Could you check a few things on this model? Use its own coordinates, in mm. Face numbers are marked on the shaded views. A direction names the side the tool comes from. Coordinates: 2 decimals unless noted, no trailing zeros. Loops run counter-clockwise (first coordinate to the right, second up) from the corner with the lowest first, then second, coordinate; pieces in that order, holes last.
1) Will this pin go through, and if not, where does the flat tip stop? P1, Ø7, axis at x = -38.5, z = -14, coming from the -Y side.
2) If I drill on line 1 along Z through (x, y) = (-44, 24); line 2 along X through (y, z) = (10, -19); line 3 along X through (y, z) = (12, 15.5), over which ranges is the centre line in solid material (lowest first)?
3) Imagine slicing it at B-B on y = 6. Give the number of separate pieces and of enclosed holes in the cut face, plus the area to 3 significant figures.
4) Imagine slicing it at C-C on x = -29.5. Please give me the cut outline in (y, z).
5) For the marked faces 1, 2 and 3, which set-ups out of +Z, -Z, +X, -X, +Y, -Y let a thin tool reach every point of the face, with its end or its side?
6) Imagine slicing it at A-A on x = -44.45. Please give me the cut outline in (y, z) (3 decimals).
7) Thinking about a two-plate mould opening in Z: for the marked faces 4, 5 and 6, which applies, released by +Z, released by -Z, zero draft, split by the parting line, or undercut?
```python
from build123d import *

# Parameters (mm, degrees)
SKETCH1_W           = 127
SKETCH1_H           = 76.2
SKETCH1_R           = 9.525
BOSS_EXTRUDE1_DEPTH = 38.1
SKETCH2_W           = 38.1
SKETCH2_H           = 76.2
CUT_EXTRUDE1_DEPTH  = 12.7
FILLET1_R           = 2.54
SHELL1_OUTLINE_W    = 121.92
SHELL1_OUTLINE_H    = 71.12
SHELL1_OUTLINE_R    = 12.065
SHELL1_DEPTH        = 22.86
SHELL1_START        = 22.86
SHELL1_2_OUTLINE_W  = 39.37
SHELL1_2_OUTLINE_H  = 71.12
SHELL1_2_OUTLINE_R  = 12.065
SHELL1_2_DEPTH      = 12.7
SHELL1_3_OUTLINE_R  = 12.065
SHELL1_3_DEPTH      = 2.54


# Read off the part's stored shape, not the designer's step: Shell1
with BuildPart() as part:
    # Sketch1 → Boss-Extrude1 (new body)
    with BuildSketch(Plane(origin=(0, 0, 0), x_dir=(1, 0, 0), z_dir=(0, 1, 0))):
        Rectangle(SKETCH1_W, SKETCH1_H)
        with Locations(Location((-44.45, 19.05, 0), (0, 0, 90))):
            Circle(SKETCH1_R, mode=Mode.SUBTRACT)
        with Locations(Location((44.45, 19.05, 0), (0, 0, 90))):
            Circle(SKETCH1_R, mode=Mode.SUBTRACT)
        with Locations(Location((-44.45, -19.05, 0), (0, 0, 90))):
            Circle(SKETCH1_R, mode=Mode.SUBTRACT)
        with Locations(Location((44.45, -19.05, 0), (0, 0, 90))):
            Circle(SKETCH1_R, mode=Mode.SUBTRACT)
    extrude(amount=BOSS_EXTRUDE1_DEPTH)

    # Sketch2 → Cut-Extrude1 (cut)
    with BuildSketch(Plane(origin=(0, 38.1, 0), x_dir=(1, 0, 0), z_dir=(0, 1, 0))):
        Rectangle(SKETCH2_W, SKETCH2_H)
    extrude(amount=-CUT_EXTRUDE1_DEPTH, mode=Mode.SUBTRACT)

    # Fillet1
    fillet1_edges = [part.edges().sort_by_distance(p)[0] for p in [
        (-44.45, 0, -9.525),
        (-44.45, 38.1, -9.525),
        (-63.5, 38.1, 0),
        (44.45, 38.1, -9.525),
        (-44.45, 38.1, 28.575),
        (44.45, 38.1, 28.575),
        (19.05, 38.1, 0),
        (-19.05, 38.1, 0),
        (63.5, 38.1, 0),
        (-63.5, 0, 0),
        (63.5, 0, 0),
    ]]
    fillet(fillet1_edges, radius=FILLET1_R)

    # Shell1 outline → Shell1 (cut)
    with BuildSketch(Plane(origin=(0, 0, 0), x_dir=(1, 0, 0), z_dir=(0, 1, 0))):
        Rectangle(SHELL1_OUTLINE_W, SHELL1_OUTLINE_H)
        with Locations((44.45, -19.05)):
            Circle(SHELL1_OUTLINE_R, mode=Mode.SUBTRACT)
        with Locations((44.45, 19.05)):
            Circle(SHELL1_OUTLINE_R, mode=Mode.SUBTRACT)
        with Locations((-44.45, 19.05)):
            Circle(SHELL1_OUTLINE_R, mode=Mode.SUBTRACT)
        with Locations((-44.45, -19.05)):
            Circle(SHELL1_OUTLINE_R, mode=Mode.SUBTRACT)
    extrude(amount=SHELL1_DEPTH, mode=Mode.SUBTRACT)

    # Shell1 2 outline → Shell1 2 (cut)
    # profile 1 of 2: a face of its own
    with BuildSketch(Plane(origin=(0, 0, 0), x_dir=(1, 0, 0), z_dir=(0, 1, 0)).offset(SHELL1_START)):
        with Locations((41.275, 0)):
            Rectangle(SHELL1_2_OUTLINE_W, SHELL1_2_OUTLINE_H)
        with Locations((44.45, -19.05)):
            Circle(SHELL1_2_OUTLINE_R, mode=Mode.SUBTRACT)
        with Locations((44.45, 19.05)):
            Circle(SHELL1_2_OUTLINE_R, mode=Mode.SUBTRACT)
    # profile 2 of 2: a face of its own
    with BuildSketch(Plane(origin=(0, 0, 0), x_dir=(1, 0, 0), z_dir=(0, 1, 0)).offset(SHELL1_START)):
        with Locations((-41.275, 0)):
            Rectangle(SHELL1_2_OUTLINE_W, SHELL1_2_OUTLINE_H)
        with Locations((-44.45, -19.05)):
            Circle(SHELL1_2_OUTLINE_R, mode=Mode.SUBTRACT)
        with Locations((-44.45, 19.05)):
            Circle(SHELL1_2_OUTLINE_R, mode=Mode.SUBTRACT)
    extrude(amount=SHELL1_2_DEPTH, mode=Mode.SUBTRACT)

    # Shell1 3 outline → Shell1 3 (cut)
    with BuildSketch(Plane(origin=(0, 0, 0), x_dir=(1, 0, 0), z_dir=(0, 1, 0))):
        with Locations((-44.45, 19.05)):
            Circle(SHELL1_3_OUTLINE_R)
    extrude(amount=SHELL1_3_DEPTH, mode=Mode.SUBTRACT)


solid = part.part
```
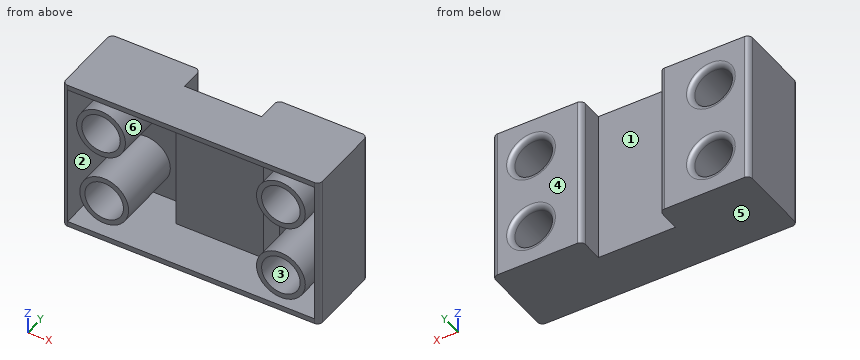
Filled in:
1. P1: stops at y = 2.54
2. line 1: z = -38.1 to -35.56, -31.11 to -28.56, -9.54 to -6.99, 6.99 to 9.54, 28.56 to 31.11, 35.56 to 38.1
2. line 2: x = -63.5 to -60.96, -56.51 to -53.97, -34.93 to -32.39, 32.39 to 34.93, 53.97 to 56.51, 60.96 to 63.5
2. line 3: x = -63.5 to -60.96, -55.98 to -53.29, -35.61 to -32.92, 32.92 to 35.61, 53.29 to 55.98, 60.96 to 63.5
3. separate pieces: 5
3. enclosed holes: 5
3. area: 1,700 mm2
4. outline: (0, -38.1) - (38.1, -38.1) - (38.1, 38.1) - (0, 38.1) - (0, 35.56) - (35.56, 35.56) - (35.56, -35.56) - (0, -35.56) - close
5. face 1: +Z, -Z, +Y
5. face 2: -Y
5. face 3: +Y, -Y
6. outline: (0, -38.1) - (38.1, -38.1) - (38.1, -31.115) arc R2.54 ccw to (35.56, -28.575) - (2.54, -28.575) - (2.54, -31.115) - (35.56, -31.115) - (35.56, -35.56) - (0, -35.56) - close; (0, 6.985) - (35.56, 6.985) - (35.56, -6.985) - (2.54, -6.985) - (2.54, -9.525) - (35.56, -9.525) arc R2.54 ccw to (38.1, -6.985) - (38.1, 6.985) arc R2.54 ccw to (35.56, 9.525) - (0, 9.525) - close; (0, 28.575) - (35.56, 28.575) arc R2.54 ccw to (38.1, 31.115) - (38.1, 38.1) - (0, 38.1) - (0, 35.56) - (35.56, 35.56) - (35.56, 31.115) - (0, 31.115) - close
7. face 4: zero draft
7. face 5: released by -Z
7. face 6: undercut
